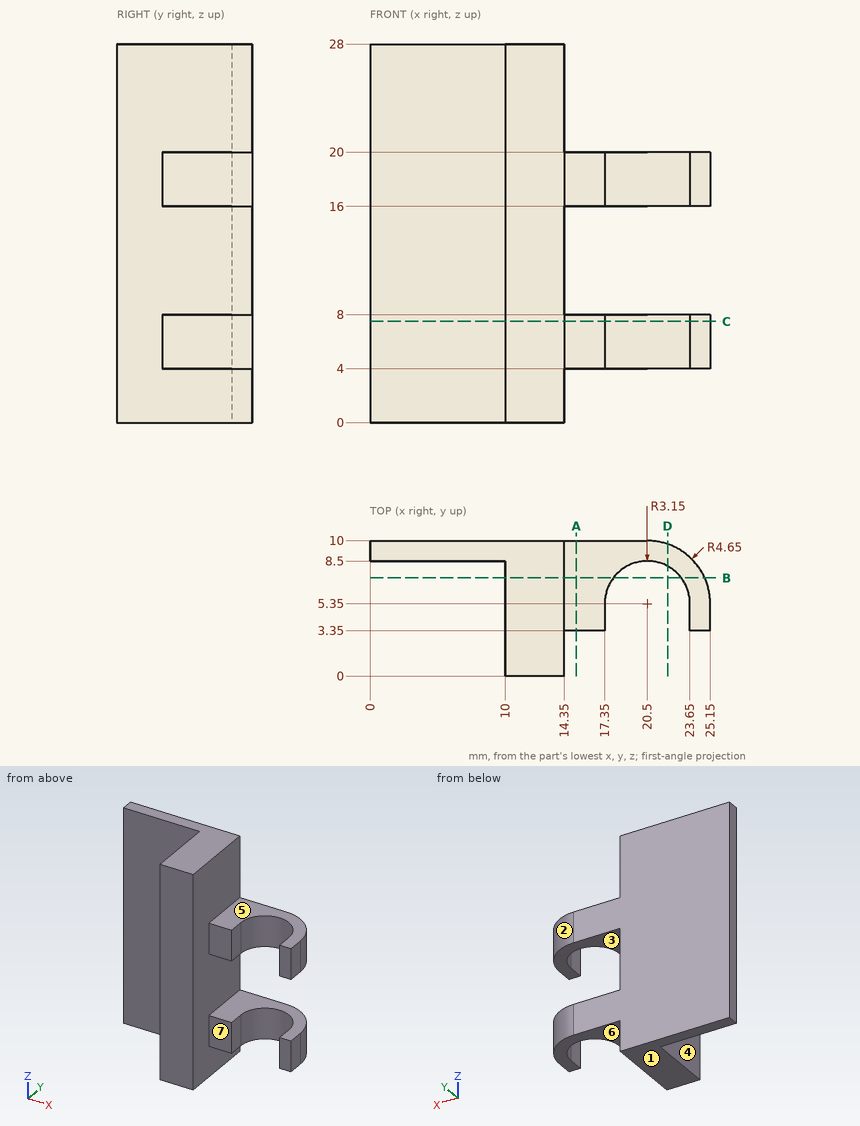
Geometry: see drawing. Coordinates: mm, zero at the bounding-box minimum. A direction names the side the tool comes from. Give positions to 0.01 mm unless a question says otherwise; leave off trailing zeros. Loops run counter-clockwise (first coordinate to the right, second up) from the corner with the lowest first, then second, coordinate; pieces in that order, holes last. Notation, with made-up numbers: (-7, 32) - (12, 32) arc R22 cw to (12, 59) - close; hole circle Ø8 at (72, 35). An arc over 180 degrees is marked (long way). Use CSV: the item, a comma, the result in double quotes. Start each with the question number.
Item 1: Section A-A on x = 15.25. Return loops of the section in (y, z), then the cut area to 3 significant figures.
Item 2: Reachability of the marked faces 4, 5, 6 and 7 from +Z, -Z, +X, -X, +Y, -Y: full face, straight path, thin tool, end or side. Return the list, or none.
Item 3: Section B-B on y = 7.25. Return loops of the section in (x, z).
Item 4: Mould query, pull axis Z, two halves, no side actions, for the marked faces 1, 2 and 3. Classes: pulls with the +Z half, pulls with the -Z half, needs draft (parallel to the pull), parting line crosses it, or undercut.
Item 5: Section C-C on z = 7.5. Return loops of the section in (x, y).
Item 6: Section D-D on x = 22. Return loops of the section in (y, z), then the cut area to 3 significant figures.
Item 7: Line query: line 1 (X direction, y = 5.5, z = 18.5); line 2 (Z direction, x = 15, y = 8.75). Output: solid intervals per line, ascending.
Item 8: Contact query for flat-ended pins moving along their axis: P1, Ø6, axis at x = 10.5, y = 3.5, coming from the -Z side; P2, Ø1.6, axis at y = 4.5, z = 6.5, coming from the -X side; P3, Ø0.9, axis at x = 15.5, z = 18, coming from the -Y side; P4, Ø3.5, axis at x = 21.5, y = 8, coming from the +Z side. Output: stop coordinate, or through.
Ans:
1,outline,"(3.35, 4) - (10, 4) - (10, 8) - (3.35, 8) - close; (3.35, 16) - (10, 16) - (10, 20) - (3.35, 20) - close"
1,area,"53.2 mm2"
2,face 4,"+Z, -Z, -X, -Y"
2,face 5,"+Z, +X, +Y, -Y"
2,face 6,"-Z, +X, +Y, -Y"
2,face 7,"+Z, -Z, +X, -Y"
3,outline,"(10, 0) - (14.35, 0) - (14.35, 4) - (17.99, 4) - (17.99, 8) - (14.35, 8) - (14.35, 16) - (17.99, 16) - (17.99, 20) - (14.35, 20) - (14.35, 28) - (10, 28) - close; (23.01, 4) - (24.74, 4) - (24.74, 8) - (23.01, 8) - close; (23.01, 16) - (24.74, 16) - (24.74, 20) - (23.01, 20) - close"
4,face 1,"pulls with the -Z half"
4,face 2,"needs draft"
4,face 3,"undercut"
5,outline,"(0, 8.5) - (10, 8.5) - (10, 0) - (14.35, 0) - (14.35, 3.35) - (17.35, 3.35) - (17.35, 5.35) arc R3.15 cw to (23.65, 5.35) - (23.65, 3.35) - (25.15, 3.35) - (25.15, 5.35) arc R4.65 ccw to (20.5, 10) - (0, 10) - close"
6,outline,"(8.12, 4) - (9.75, 4) - (9.75, 8) - (8.12, 8) - close; (8.12, 16) - (9.75, 16) - (9.75, 20) - (8.12, 20) - close"
6,area,"13.1 mm2"
7,line 1,"x = 10 to 17.35, 23.65 to 25.15"
7,line 2,"z = 4 to 8, 16 to 20"
8,P1,"stops at z = 0"
8,P2,"stops at x = 10"
8,P3,"stops at y = 3.35"
8,P4,"stops at z = 20"
